```python
from build123d import *

# Parameters (mm, degrees)
SKETCH1_W                    = 68
SKETCH1_H                    = 42
BOSS_EXTRUDE1_DEPTH          = 1
SKETCH3_W                    = 1
SKETCH3_H                    = 42
EXTRUDE_THIN1_DEPTH          = 20
SKETCH4_R                    = 5
CUT_EXTRUDE1_DEPTH           = 144.394560566
SKETCH6_W                    = 3
SKETCH6_H                    = 11
CUT_EXTRUDE2_DEPTH           = 143.779550356
SKETCH6_3_R                  = 4
BOSS_EXTRUDE2_DEPTH          = 15
SKETCH6_4_R                  = 2.5
SKETCH6_4_R_2                = 4
BOSS_EXTRUDE3_DEPTH          = 6
SKETCH7_W                    = 1
SKETCH7_H                    = 42
BOSS_EXTRUDE5_DEPTH          = 1
FILLET2_R                    = 5
SKETCH8_W                    = 60
SKETCH8_H                    = 1
BOSS_EXTRUDE6_DEPTH          = 20
CONVERT_SOLID1_START         = -20
CONVERT_SOLID1_OUTLINE_W     = 1
CONVERT_SOLID1_OUTLINE_H     = 42
CONVERT_SOLID1_OUTLINE_W_2   = 60
CONVERT_SOLID1_OUTLINE_H_2   = 1
CONVERT_SOLID1_DEPTH         = 20
CONVERT_SOLID1_2_OUTLINE_R   = 2.5
CONVERT_SOLID1_2_OUTLINE_R_2 = 4
CONVERT_SOLID1_2_DEPTH       = 16


# Read off the part's stored shape, not the designer's step: Convert-Solid1
with BuildPart() as part:
    # Sketch1 → Boss-Extrude1 (new body)
    with BuildSketch(Plane.XY):
        Polygon((-38, 62), (-38, 42), (0, 42), (68, 42), (108, 42), (108, 67), (65, 78), (65, 91), (5, 91), (5, 78), align=None)
        with Locations((34, 21)):
            Rectangle(SKETCH1_W, SKETCH1_H)
    extrude(amount=BOSS_EXTRUDE1_DEPTH)

    # Sketch3 → Extrude-Thin1 (add)
    with BuildSketch(Plane(origin=(0, 0, 0), x_dir=(-1, 0, 0), z_dir=(0, 0, -1))):
        with Locations((0.5, 21)):
            Rectangle(SKETCH3_W, SKETCH3_H)
        with Locations((-67.5, 21)):
            Rectangle(SKETCH3_W, SKETCH3_H)
    extrude(amount=EXTRUDE_THIN1_DEPTH)


with BuildPart() as extrude_thin1_piece_1:
    # of the separate pieces the step leaves, piece 1, a body of its own (extrude_thin1_pieces)
    add(part.part.solids().sort_by_distance((-38, 62, 0))[0])


with BuildPart() as extrude_thin1_piece_2:
    # of the separate pieces the step leaves, piece 2, a body of its own (extrude_thin1_pieces)
    add(part.part.solids().sort_by_distance((0, 42, -20))[0])


with BuildPart() as cut_extrude1_tool:
    # Sketch4 → Cut-Extrude1 (new, through all)
    with BuildSketch(Plane.ZY.offset(1)):
        with Locations((-9.5, 15)):
            Circle(SKETCH4_R)
    extrude(amount=-CUT_EXTRUDE1_DEPTH)


with BuildPart() as extrude_thin1_piece_1_1:
    add(extrude_thin1_piece_1.part)

    # Cut-Extrude1: cut by cut_extrude1_tool
    add(cut_extrude1_tool.part, mode=Mode.SUBTRACT)

    # Sketch6 → Cut-Extrude2 (cut, through all)
    with BuildSketch(Plane.XY.offset(1)):
        with Locations((100.5, 56.5)):
            Rectangle(SKETCH6_W, SKETCH6_H)
        with Locations((-30.5, 51)):
            Rectangle(SKETCH6_W, SKETCH6_H)
        with BuildLine():
            Line((49.095389312, 77.86969785), (44.396926208, 79.579798567))
            ThreePointArc((44.396926208, 79.579798567), (35, 73), (25.603073792, 79.579798567))
            Line((25.603073792, 79.579798567), (20.904610688, 77.86969785))
            ThreePointArc((20.904610688, 77.86969785), (35, 68), (49.095389312, 77.86969785))
        make_face()
    extrude(amount=-CUT_EXTRUDE2_DEPTH, mode=Mode.SUBTRACT)

    # Sketch6<3> → Boss-Extrude2 (add)
    with BuildSketch(Plane.XY.offset(1)):
        with Locations((35, 83)):
            Circle(SKETCH6_3_R)
    extrude(amount=BOSS_EXTRUDE2_DEPTH)

    # Sketch6<4> → Boss-Extrude3 (add)
    with BuildSketch(Plane.XY.offset(1)):
        with Locations((35, 10)):
            Circle(SKETCH6_4_R)
        with Locations((35, 25)):
            Circle(SKETCH6_4_R_2)
    extrude(amount=BOSS_EXTRUDE3_DEPTH)



with BuildPart() as extrude_thin1_piece_2_1:
    add(extrude_thin1_piece_2.part)

    # Cut-Extrude1: cut by cut_extrude1_tool
    add(cut_extrude1_tool.part, mode=Mode.SUBTRACT)


with BuildPart() as extrude_thin1_piece_1_2:
    add(extrude_thin1_piece_1_1.part)

    add(extrude_thin1_piece_2_1.part)  # Boss-Extrude5 merges Extrude-Thin1 piece 2
    # Sketch7 → Boss-Extrude5 (add)
    with BuildSketch(Plane.XY):
        with Locations((-0.5, 21)):
            Rectangle(SKETCH7_W, SKETCH7_H)
    extrude(amount=BOSS_EXTRUDE5_DEPTH)

    # Fillet2
    fillet2_edges = [extrude_thin1_piece_1_2.edges().sort_by_distance(p)[0] for p in [
        (-0.5, 0, -20),
        (-38, 42, 0.5),
        (-38, 62, 0.5),
        (67.5, 0, -20),
        (108, 42, 0.5),
        (108, 67, 0.5),
        (67.5, 42, -20),
        (-0.5, 42, -20),
    ]]
    fillet(fillet2_edges, radius=FILLET2_R)

    # Sketch8 → Boss-Extrude6 (add)
    with BuildSketch(Plane(origin=(0, 0, 0), x_dir=(-1, 0, 0), z_dir=(0, 0, -1))):
        with Locations((-35, 90.5)):
            Rectangle(SKETCH8_W, SKETCH8_H)
    extrude(amount=BOSS_EXTRUDE6_DEPTH)

    # Convert-Solid1 outline → Convert-Solid1 (cut)
    with BuildSketch(Plane.XY.offset(CONVERT_SOLID1_START)):
        with Locations((-0.5, 21)):
            Rectangle(CONVERT_SOLID1_OUTLINE_W, CONVERT_SOLID1_OUTLINE_H)
        with Locations((67.5, 21)):
            Rectangle(CONVERT_SOLID1_OUTLINE_W, CONVERT_SOLID1_OUTLINE_H)
        with Locations((35, 90.5)):
            Rectangle(CONVERT_SOLID1_OUTLINE_W_2, CONVERT_SOLID1_OUTLINE_H_2)
    extrude(amount=CONVERT_SOLID1_DEPTH, mode=Mode.SUBTRACT)

    # Convert-Solid1 2 outline → Convert-Solid1 2 (cut)
    with BuildSketch(Plane.XY):
        with Locations((35, 10)):
            Circle(CONVERT_SOLID1_2_OUTLINE_R)
        with Locations((35, 25)):
            Circle(CONVERT_SOLID1_2_OUTLINE_R_2)
        with Locations((35, 83)):
            Circle(CONVERT_SOLID1_2_OUTLINE_R_2)
    extrude(amount=CONVERT_SOLID1_2_DEPTH, mode=Mode.SUBTRACT)


solid = extrude_thin1_piece_1_2.part
```
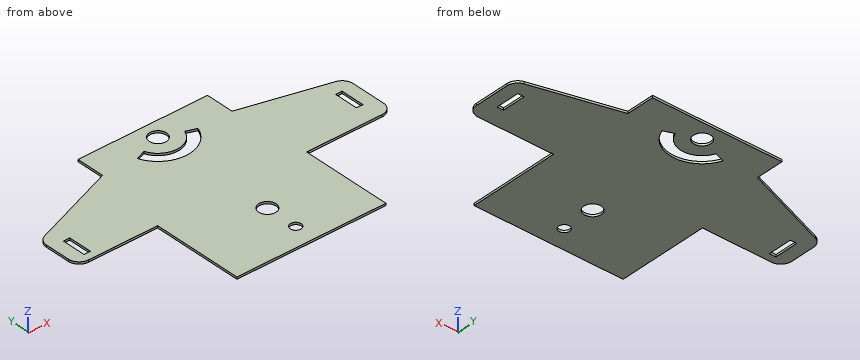
Geometry: final body of the model. Coordinates: model frame, mm. Coordinates: 2 decimals unless noted, no trailing zeros. Order: outer loops, then holes, each group sorted by start corner. A loop starts at its lowest first (then second) coordinate and runs counter-clockwise, first axis right, second up. Notation, with made-up numbers: (47, 60.25) - (101, 60.25) arc R27 cw to (101, 78.25) - close; hole circle Ø1 at (40.25, 29). An arc over 180 degrees is marked (long way). Write each question's results on one line, items separated by ' | '.
1) Section D-D, the plane y = 83. Return loops of the section in (x, z).
Results list:
outline: (5, 0) - (31, 0) - (31, 1) - (5, 1) - close; (39, 0) - (65, 0) - (65, 1) - (39, 1) - close
2) Line query: line 1 (Y direction, x = 35, z = 0.3); line 2 (X direction, y = 47.5, z = 0.5); line 3 (Y direction, x = 22, z = 0.2). Output: solid intervals per line, ascending. Write a range as from..to.
Results list:
line 1: 0..7.5, 12.5..21, 29..68, 73..79, 87..91 | line 2: -38..-32, -29..108 | line 3: 0..75.52, 78.27..91
3) Pin query (flat end, axial travel): pin 1 (0.5 mm diameter, centred on x = -31, z = 0.5, fed in from +Y). Return the tip coordinate at first contact, or that it passes through.
Results list:
pin 1: y = 64.7
4) Section A-A, the plane x = 35. Return loops of the section in (y, z), plus the area to 3 significant figures.
Results list:
outline: (0, 0) - (7.5, 0) - (7.5, 1) - (0, 1) - close; (12.5, 0) - (21, 0) - (21, 1) - (12.5, 1) - close; (29, 0) - (68, 0) - (68, 1) - (29, 1) - close; (73, 0) - (79, 0) - (79, 1) - (73, 1) - close; (87, 0) - (91, 0) - (91, 1) - (87, 1) - close | area: 65.0 mm^2
5) Section B-B, the plane z = 0.15. State how many separate pieces and enclosed holes the cut face has, plus the area to 3 significant figures.
Results list:
separate pieces: 1 | enclosed holes: 6 | area: 8,000 mm^2
6) Section C-C, the plane y = 10. Return loops of the section in (x, z), plus the area to 3 significant figures.
Results list:
outline: (-1, 0) - (32.5, 0) - (32.5, 1) - (-1, 1) - close; (37.5, 0) - (68, 0) - (68, 1) - (37.5, 1) - close | area: 64.0 mm^2
